```python
from build123d import *

# Parameters (mm, degrees)
SK_P01_STANDOFF_R                  = 2.5
P01_STANDOFF_DEPTH                 = 6
SK_P02_STANDOFF_R                  = 2.5
P02_STANDOFF_DEPTH                 = 6
SK_P03_STANDOFF_R                  = 2.5
P03_STANDOFF_DEPTH                 = 6
SK_P04_STANDOFF_R                  = 2.5
P04_STANDOFF_DEPTH                 = 6
P05_DFR0601BOARD50X50_START        = 6
SK_P05_DFR0601BOARD50X50_W         = 50
SK_P05_DFR0601BOARD50X50_H         = 50
P05_DFR0601BOARD50X50_DEPTH        = 1.6
P06_MOSFETSANDHEATSINK_START       = 7.6
SK_P06_MOSFETSANDHEATSINK_W        = 26
SK_P06_MOSFETSANDHEATSINK_H        = 34
P06_MOSFETSANDHEATSINK_DEPTH       = 10.9
P07_POWERANDMOTORTERMINALSWI_START = 7.6
SK_P07_POWERANDMOTORTERMINALSWI_W  = 9
SK_P07_POWERANDMOTORTERMINALSWI_H  = 46
P07_POWERANDMOTORTERMINALSWI_DEPTH = 10.9
P08_CONTROLHEADER_START            = 7.6
SK_P08_CONTROLHEADER_W             = 7
SK_P08_CONTROLHEADER_H             = 20
P08_CONTROLHEADER_DEPTH            = 8.4


with BuildPart() as part:
    # SK_P01_Standoff → P01_Standoff (new body)
    with BuildSketch(Plane(origin=(0, 0, 0), x_dir=(1, 0, 0), z_dir=(0, 1, 0))):
        with Locations(Location((-20, 20, 0), (0, 0, 270))):
            Circle(SK_P01_STANDOFF_R)
    extrude(amount=P01_STANDOFF_DEPTH)



with BuildPart() as body_2:
    # SK_P02_Standoff → P02_Standoff (new body)
    with BuildSketch(Plane(origin=(0, 0, 0), x_dir=(1, 0, 0), z_dir=(0, 1, 0))):
        with Locations(Location((20, 20, 0), (0, 0, 270))):
            Circle(SK_P02_STANDOFF_R)
    extrude(amount=P02_STANDOFF_DEPTH)


with BuildPart() as body_3:
    # SK_P03_Standoff → P03_Standoff (new body)
    with BuildSketch(Plane(origin=(0, 0, 0), x_dir=(1, 0, 0), z_dir=(0, 1, 0))):
        with Locations(Location((-20, -20, 0), (0, 0, 270))):
            Circle(SK_P03_STANDOFF_R)
    extrude(amount=P03_STANDOFF_DEPTH)


with BuildPart() as body_4:
    # SK_P04_Standoff → P04_Standoff (new body)
    with BuildSketch(Plane(origin=(0, 0, 0), x_dir=(1, 0, 0), z_dir=(0, 1, 0))):
        with Locations(Location((20, -20, 0), (0, 0, 270))):
            Circle(SK_P04_STANDOFF_R)
    extrude(amount=P04_STANDOFF_DEPTH)


with BuildPart() as part_1:
    add(part.part)

    add(body_2.part)  # P05_DFR0601board50x50 merges body 2

    add(body_3.part)  # P05_DFR0601board50x50 merges body 3

    add(body_4.part)  # P05_DFR0601board50x50 merges body 4
    # SK_P05_DFR0601board50x50 → P05_DFR0601board50x50 (add)
    with BuildSketch(Plane(origin=(0, 0, 0), x_dir=(1, 0, 0), z_dir=(0, 1, 0)).offset(P05_DFR0601BOARD50X50_START)):
        Rectangle(SK_P05_DFR0601BOARD50X50_W, SK_P05_DFR0601BOARD50X50_H)
    extrude(amount=P05_DFR0601BOARD50X50_DEPTH)

    # SK_P06_MOSFETsandheatsink → P06_MOSFETsandheatsink (add)
    with BuildSketch(Plane(origin=(0, 0, 0), x_dir=(1, 0, 0), z_dir=(0, 1, 0)).offset(P06_MOSFETSANDHEATSINK_START)):
        Rectangle(SK_P06_MOSFETSANDHEATSINK_W, SK_P06_MOSFETSANDHEATSINK_H)
    extrude(amount=P06_MOSFETSANDHEATSINK_DEPTH)

    # SK_P07_Powerandmotorterminalswi → P07_Powerandmotorterminalswi (add)
    with BuildSketch(Plane(origin=(0, 0, 0), x_dir=(1, 0, 0), z_dir=(0, 1, 0)).offset(P07_POWERANDMOTORTERMINALSWI_START)):
        with Locations((20.5, 0)):
            Rectangle(SK_P07_POWERANDMOTORTERMINALSWI_W, SK_P07_POWERANDMOTORTERMINALSWI_H)
    extrude(amount=P07_POWERANDMOTORTERMINALSWI_DEPTH)

    # SK_P08_Controlheader → P08_Controlheader (add)
    with BuildSketch(Plane(origin=(0, 0, 0), x_dir=(1, 0, 0), z_dir=(0, 1, 0)).offset(P08_CONTROLHEADER_START)):
        with Locations((-19.5, 7)):
            Rectangle(SK_P08_CONTROLHEADER_W, SK_P08_CONTROLHEADER_H)
    extrude(amount=P08_CONTROLHEADER_DEPTH)


solid = part_1.part
```
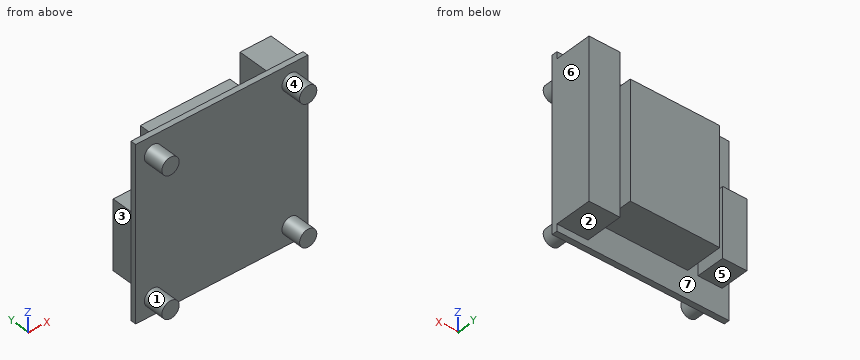
CAD build for the part. Positions are in the model's coordinates, mm. Face numbers are marked on the shaded views. A direction names the side the tool comes from. Coordinates: 2 decimals unless noted, no trailing zeros. Write each loop counter-clockwise with the first axis right and the second up, starting at its lowest first coordinate (ties: lowest second). Pieces come first, ordered by that corner, then holes. Notation, with made-up numbers: (33.25, 83) -> (69.25, 83) arc R25 ccw to (69.25, 97) -> close; hole circle Ø8 at (45, 63). An arc over 180 degrees is marked (long way). Return JSON: item names as keys, results as strings. Group by question number.
Q1. Which spindle directions (+Z, -Z, +X, -X, +Y, -Y) get a long thin tool onto all of the face, cutting with end or side? Do the marked faces 1, 2 and 3. Say none if no direction does.
Q2. Cut at A-A, the plane y = 11.75. Give the cut face in (x, z), then the cut area to 3 significant figures.
Q3. Flat gauge pins, fed straight in: pin 1 (25 mm diameter, centred on x = 12, z = 5, fed in from -Y); pin 2 (1.5 mm diameter, centred on y = 3, z = 17, fed in from -X); pin 3 (4 mm diameter, centred on y = 2.5, z = -18, fed in from +X). Where does each tip first touch, or does it go through?
Q4. Cut at D-D, the plane z = 12. Give the cut face in (x, y), then the cut area to 4 significant figures.
Q5. Drill centre lines: line 1 (X direction, y = 10, z = -3.5); line 2 (X direction, y = 17.5, z = -14.5); line 3 (X direction, y = 12.5, z = 21.5). Where is each one in solid material? Low to high.
Q6. Cut at C-C, the plane x = 20. Give the cut face in (y, z).
Q7. Cut at B-B, the plane y = 17. Give the cut face in (x, z), then the cut area to 3 significant figures.
Q8. Pull direction X, two halves, no side cores. Call the marked faces 4, 5, 6 and 7: released by +X, released by -X, zero draft, split by the parting line, or undercut.
Returned:
{
 "1": {"face 1": "-Y", "face 2": "-Z, +X, -X, +Y", "face 3": "+Z, -Z, -X, +Y"},
 "2": {"outline": "(-23, -17) -> (-16, -17) -> (-16, 3) -> (-23, 3) -> close; (-13, -17) -> (13, -17) -> (13, 17) -> (-13, 17) -> close; (16, -23) -> (25, -23) -> (25, 23) -> (16, 23) -> close", "area": "1,440 mm2"},
 "3": {"pin 1": "stops at y = 6", "pin 2": "stops at x = -21.09", "pin 3": "stops at x = 22.5"},
 "4": {"outline": "(-25, 6) -> (25, 6) -> (25, 18.5) -> (16, 18.5) -> (16, 7.6) -> (13, 7.6) -> (13, 18.5) -> (-13, 18.5) -> (-13, 7.6) -> (-25, 7.6) -> close", "area": "461.5 mm2"},
 "5": {"line 1": "x = -23 to -16, -13 to 13, 16 to 25", "line 2": "x = -13 to 13, 16 to 25", "line 3": "x = 16 to 25"},
 "6": {"outline": "(0, -22.5) -> (6, -22.5) -> (6, -25) -> (7.6, -25) -> (7.6, -23) -> (18.5, -23) -> (18.5, 23) -> (7.6, 23) -> (7.6, 25) -> (6, 25) -> (6, 22.5) -> (0, 22.5) -> (0, 17.5) -> (6, 17.5) -> (6, -17.5) -> (0, -17.5) -> close"},
 "7": {"outline": "(-13, -17) -> (13, -17) -> (13, 17) -> (-13, 17) -> close; (16, -23) -> (25, -23) -> (25, 23) -> (16, 23) -> close", "area": "1,300 mm2"},
 "8": {"face 4": "undercut", "face 5": "zero draft", "face 6": "released by +X", "face 7": "undercut"}
}
